Read the model definition and answer for the solid it produces. Units are mm, in the model's axes. Face numbers are marked on the shaded views. A direction names the side the tool comes from. Give positions to 0.01 mm unless a question says otherwise; leave off trailing zeros. Loops run counter-clockwise (first coordinate to the right, second up) from the corner with the lowest first, then second, coordinate; pieces in that order, holes last. Notation, with made-up numbers: (55.25, 44) -> (66.25, 44) arc R22 ccw to (66.25, 69) -> close; hole circle Ø11 at (46.5, 21.5). An arc over 180 degrees is marked (long way). Return JSON: item names as keys, results as strings. Group by question number.
from build123d import *

# Parameters (mm, degrees)
SKETCH_1_W             = 29.1
SKETCH_1_H             = 6.5
EXTRUDE_1_DEPTH        = 5
EXTRUDE_2_DEPTH        = 8
SKETCH_3_R             = 3
CUT_EXTRUDE_1118_DEPTH = 3
EXTRUDE_1407_DEPTH     = 6
SKETCH_5_R             = 1.25
CUT_EXTRUDE_2_DEPTH    = 38.469587668
CHAMFER_1_SIZE         = 1
SKETCH_6_R             = 1.087134162
CUT_EXTRUDE_3_DEPTH    = 5
CHAMFER_2_SIZE         = 1
SKETCH_7_R             = 1.482090692
CUT_EXTRUDE_4_DEPTH    = 5
CHAMFER_3_SIZE         = 1


with BuildPart() as part:
    # Эскиз1 → Бобышка-Вытянуть1 (new body)
    with BuildSketch(Plane.XY):
        with Locations((-14.55, 3.25)):
            Rectangle(SKETCH_1_W, SKETCH_1_H)
    extrude(amount=EXTRUDE_1_DEPTH)

    # Эскиз2 → Бобышка-Вытянуть2 (add)
    with BuildSketch(Plane(origin=(0, 0, 0), x_dir=(-1, 0, 0), z_dir=(0, 0, -1))):
        Polygon((0, -8.6), (-2, -8.6), (-2, -10.6), (31.1, -10.6), (31.1, -8.6), (29.1, -8.6), align=None)
        Polygon((0, 0), (0, 6.5), (-2, 6.5), (-2, -8.6), (0, -8.6), align=None)
        Polygon((29.1, 0), (29.1, -8.6), (31.1, -8.6), (31.1, 6.5), (29.1, 6.5), align=None)
    extrude(amount=-EXTRUDE_2_DEPTH)

    # Эскиз3 → Cut-Extrude 1118 (cut)
    with BuildSketch(Plane(origin=(2, 0, 0), x_dir=(0, 0, -1), z_dir=(1, 0, 0))):
        with Locations((-8, -4.6)):
            Circle(SKETCH_3_R)
    extrude(amount=-CUT_EXTRUDE_1118_DEPTH, mode=Mode.SUBTRACT)

    # Эскиз4 → Extrude 1407 (add)
    with BuildSketch(Plane.XY.offset(8)):
        Polygon((2, 6.5), (2, -10.6), (-31.1, -10.6), (-31.1, 6.5), (-29.1, 6.5), (-29.1, -8.6), (0, -8.6), (0, 6.5), align=None)
    extrude(amount=EXTRUDE_1407_DEPTH)

    # Эскиз5 → Вырез-Вытянуть2 (cut, through all)
    with BuildSketch(Plane(origin=(2, 0, 0), x_dir=(0, 0, -1), z_dir=(1, 0, 0))):
        with Locations(Location((-11, -2.05, 0), (0, 0, 90))):
            Circle(SKETCH_5_R)
    extrude(amount=-CUT_EXTRUDE_2_DEPTH, mode=Mode.SUBTRACT)

    # Фаска1
    chamfer_1_edges = [part.edges().sort_by_distance(p)[0] for p in [
        (-31.1, -3.3, 11),
        (2, -3.3, 11),
    ]]
    chamfer(chamfer_1_edges, length=CHAMFER_1_SIZE)

    # Эскиз6 → Вырез-Вытянуть3 (cut)
    with BuildSketch(Plane(origin=(0, -10.6, 0), x_dir=(-1, 0, 0), z_dir=(0, -1, 0))):
        with Locations(Location((14.55, -11, 0), (0, 0, 90))):
            Circle(SKETCH_6_R)
    extrude(amount=-CUT_EXTRUDE_3_DEPTH, mode=Mode.SUBTRACT)

    # Фаска2
    chamfer_2_edges = [part.edges().sort_by_distance(p)[0] for p in [
        (-14.55, -10.6, 12.087134162),
    ]]
    chamfer(chamfer_2_edges, length=CHAMFER_2_SIZE)

    # Эскиз7 → Вырез-Вытянуть4 (cut)
    with BuildSketch(Plane(origin=(0, 0, 0), x_dir=(-1, 0, 0), z_dir=(0, 0, -1))):
        with Locations((14.290801776, 3.5)):
            Circle(SKETCH_7_R)
    extrude(amount=-CUT_EXTRUDE_4_DEPTH, mode=Mode.SUBTRACT)

    # Фаска3
    chamfer_3_edges = [part.edges().sort_by_distance(p)[0] for p in [
        (-12.808711084, 3.5, 0),
    ]]
    chamfer(chamfer_3_edges, length=CHAMFER_3_SIZE)


solid = part.part
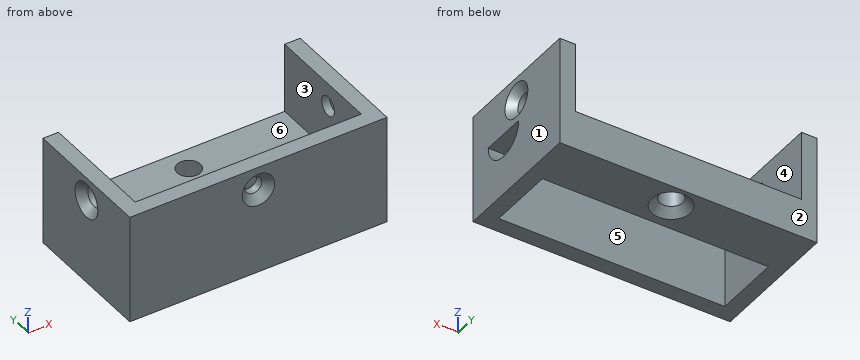
1. Determine the mould class of the marked faces 1, 2 and 3 for opening direction Y: pulls with the +Y half, pulls with the -Y half, needs draft (parallel to the pull), parting line crosses it, or undercut.
2. Section A-A on x = -11 is taken. Determine the outline of the cut face in (y, z), then the cut area to 3 significant figures.
3. Section D-D on z = 7 is taken. Determine the outline of the cut face in (x, y), then the cut area to 3 significant figures.
4. Flat-ended cylindrical pins translate along their axes: pin 1 Ø5 at (x, y) = (-8.5, 5) entering from +Z; pin 2 Ø3 at (y, z) = (-2.05, 11) entering from -X; pin 3 Ø4.5 at (x, y) = (-14.29, 3.5) entering from -Z. Find the tip coordinate at first contact, or state that the pin passes through.
5. Section B-B on y = -8 is taken. Determine the outline of the cut face in (x, z), then the cut area to 3 significant figures.
6. Section C-C on z = 11 is taken. Determine the outline of the cut face in (x, y).
7. Straight lines are drawn through the part: line 1 (X direction, y = -7.5, z = 6.5); line 2 (Y direction, x = -28, z = 4); line 3 (Z direction, x = -29.3, y = -2.05). For each, find the intervals that lie inside material, in ascending order. Write a range as from..to.
8. Which of the six approach directions +Z, -Z, +X, -X, +Y, -Y give full straight-line access (tool end or side, diameter ignored) to the marked faces 4, 5 and 6?
Completed:
{
 "1": {"face 1": "needs draft", "face 2": "pulls with the +Y half", "face 3": "undercut"},
 "2": {"outline": "(-10.6, 0) -> (-8.6, 0) -> (-8.6, 14) -> (-10.6, 14) -> close; (0, 0) -> (6.5, 0) -> (6.5, 5) -> (0, 5) -> close", "area": "60.5 mm²"},
 "3": {"outline": "(-31.1, -10.6) -> (2, -10.6) -> (2, -7.43) -> (0, -7.43) -> (0, -8.6) -> (-29.1, -8.6) -> (-29.1, 6.5) -> (-31.1, 6.5) -> close; (0, -1.77) -> (2, -1.77) -> (2, 6.5) -> (0, 6.5) -> close", "area": "115 mm²"},
 "4": {"pin 1": "stops at z = 5", "pin 2": "stops at x = -30.35", "pin 3": "stops at z = 0.23"},
 "5": {"outline": "(-31.1, 0) -> (-29.1, 0) -> (-29.1, 14) -> (-31.1, 14) -> close; (0, 0) -> (2, 0) -> (2, 14) -> (0, 14) -> close", "area": "56.0 mm²"},
 "6": {"outline": "(-31.1, -10.6) -> (-16.64, -10.6) -> (-15.64, -9.6) -> (-15.64, -8.6) -> (-29.1, -8.6) -> (-29.1, -3.3) -> (-30.1, -3.3) -> (-31.1, -4.3) -> close; (-31.1, 0.2) -> (-30.1, -0.8) -> (-29.1, -0.8) -> (-29.1, 6.5) -> (-31.1, 6.5) -> close; (-13.46, -9.6) -> (-12.46, -10.6) -> (2, -10.6) -> (2, -4.3) -> (1, -3.3) -> (0, -3.3) -> (0, -8.6) -> (-13.46, -8.6) -> close; (0, -0.8) -> (1, -0.8) -> (2, 0.2) -> (2, 6.5) -> (0, 6.5) -> close"},
 "7": {"line 1": "x = -31.1..-29.1, 0..2", "line 2": "y = -10.6..-8.6, 0..6.5", "line 3": "z = 0..9.75, 12.25..14"},
 "8": {"face 4": "+Z", "face 5": "+Z, -Z", "face 6": "+Z, +Y"}
}
